Study the drawing (mm; zero at the part's minimum x, y, z) and answer. Round coordinates to 2 decimals unless told otherwise and drop trailing zeros. Write each loop counter-clockwise with the first axis right and the second up, starting at its lowest first coordinate (ties: lowest second). Pieces come first, ordered by that corner, then holes. Notation, with made-up numbers: (76.25, 18) - (94.25, 18) arc R10 cw to (94.25, 34) - close; hole circle Ø5 at (41.25, 59.25). An arc over 180 degrees is marked (long way). Return JSON: item names as keys, results as strings. Group by question number.
(1) Find the intervals of material crossed by line 1 along Y through (x, z) = (5.9, 0.8); line 2 along X through (y, z) = (40, 0.7); line 3 along X through (y, z) = (22, 0.8), in increasing order. Write a range as [from, to].
(2) Section D-D, the plane z = 0.6 is taken. Write down the section's boundary in (x, y), then the cut area to 3 significant figures.
(3) Section C-C, the plane y = 29.5 is taken. Write down the section's boundary in (x, z).
(4) This flat-tipped pin is pushed along its axis until it touches: pin 1 (3.5 mm diameter, centred on x = 5.9, y = 53.1, fed in from -Z). Where does it stop, or does it pass through?
(5) Section A-A, the plane y = 5.9 is taken. Write down the section's boundary in (x, z), then the cut area to 3 significant figures.
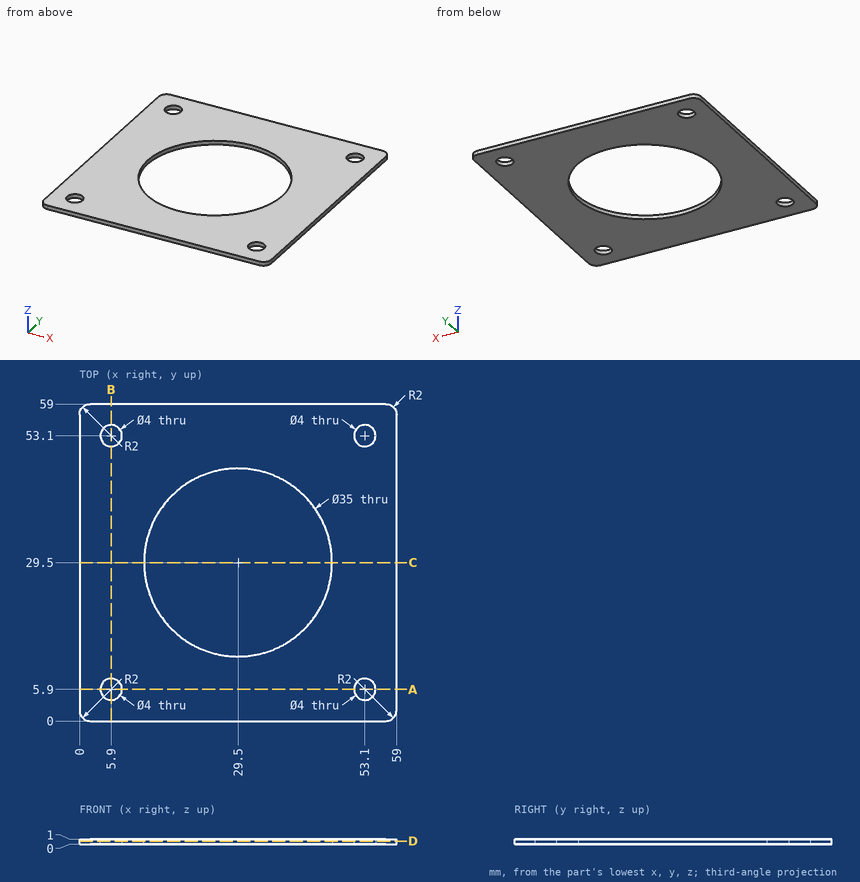
Working result:
{
 "1": {"line 1": "y = [0, 3.9], [7.9, 51.1], [55.1, 59]", "line 2": "x = [0, 15.5], [43.5, 59]", "line 3": "x = [0, 13.69], [45.31, 59]"},
 "2": {"outline": "(0, 2) arc R2 ccw to (2, 0) - (57, 0) arc R2 ccw to (59, 2) - (59, 57) arc R2 ccw to (57, 59) - (2, 59) arc R2 ccw to (0, 57) - close; hole circle Ø4 at (5.9, 5.9); hole circle Ø4 at (5.9, 53.1); hole circle Ø35 at (29.5, 29.5); hole circle Ø4 at (53.1, 5.9); hole circle Ø4 at (53.1, 53.1)", "area": "2,470 mm^2"},
 "3": {"outline": "(0, 0) - (12, 0) - (12, 1) - (0, 1) - close; (47, 0) - (59, 0) - (59, 1) - (47, 1) - close"},
 "4": {"pin 1": "passes through"},
 "5": {"outline": "(0, 0) - (3.9, 0) - (3.9, 1) - (0, 1) - close; (7.9, 0) - (51.1, 0) - (51.1, 1) - (7.9, 1) - close; (55.1, 0) - (59, 0) - (59, 1) - (55.1, 1) - close", "area": "51.0 mm^2"}
}
